```python
from build123d import *

# Parameters (mm, degrees)
F0_W     = 127
F0_H     = 152.4
F0_W_2   = 103
F0_H_2   = 64.5
F1_DEPTH = 6
F2_DEPTH = 2
F3_R     = 3.175


with BuildPart() as f1:
    # F0 (on Top) → F1 (new body)
    with BuildSketch(Plane.XY):
        Rectangle(F0_W, F0_H)
        Rectangle(F0_W_2, F0_H_2, mode=Mode.SUBTRACT)
        Rectangle(F0_W_2, F0_H_2)
    extrude(amount=F1_DEPTH)

    # F0 (on Top) → F2 (cut)
    with BuildSketch(Plane.XY):
        Rectangle(F0_W_2, F0_H_2)
    extrude(amount=F2_DEPTH, mode=Mode.SUBTRACT)

    # F3
    f3_edges = [f1.edges().sort_by_distance(p)[0] for p in [
        (63.5, -76.2, 3),
        (-63.5, -76.2, 3),
        (63.5, 76.2, 3),
        (-63.5, 76.2, 3),
    ]]
    fillet(f3_edges, radius=F3_R)


solid = f1.part
```
Input: part model. Units: mm. Frame: model coordinates. Give positions to 0.01 mm unless a question says otherwise; leave off trailing zeros. Order: outer loops, then holes, each group sorted by start corner. A loop starts at its lowest first (then second) coordinate and runs counter-clockwise, first axis right, second up.
1. Section A-A on z = 1.1. Return the cut outline in (x, y) (3 decimals).
Derived:
outline: (-63.5, -73.025) arc R3.175 ccw to (-60.325, -76.2) - (60.325, -76.2) arc R3.175 ccw to (63.5, -73.025) - (63.5, 73.025) arc R3.175 ccw to (60.325, 76.2) - (-60.325, 76.2) arc R3.175 ccw to (-63.5, 73.025) - close; hole (-51.5, -32.25) - (51.5, -32.25) - (51.5, 32.25) - (-51.5, 32.25) - close
2. Material intervals for L1, parallel to Y at x = -7.5, z = 0.45; L2, parallel to X at y = 29, z = 0.45; L3, parallel to Z at x = -2, y = -12.5, sorted ascending.
Derived:
L1: y = -76.2 to -32.25, 32.25 to 76.2
L2: x = -63.5 to -51.5, 51.5 to 63.5
L3: z = 2 to 6
3. Section B-B on y = -6.5. Return the cut outline in (x, z).
Derived:
outline: (-63.5, 0) - (-51.5, 0) - (-51.5, 2) - (51.5, 2) - (51.5, 0) - (63.5, 0) - (63.5, 6) - (-63.5, 6) - close
4. Mould query, pull axis Y, two halves, no side actions, for faces 1 (the flat face through (-1, 1, 6)), 2 (the flat face through (-1, 76.2, 3)), 3 (the cylindrical face through (62.55, -75.29, 3.04)), 4 (the flat face through (-1, 0, 2)). Classes: released by +Y, released by -Y, zero draft, split by the parting line, or undercut.
Derived:
face 1: zero draft
face 2: released by +Y
face 3: released by -Y
face 4: undercut
5. Section C-C on x = -48. Return the cut outline in (y, z).
Derived:
outline: (-76.2, 0) - (-32.25, 0) - (-32.25, 2) - (32.25, 2) - (32.25, 0) - (76.2, 0) - (76.2, 6) - (-76.2, 6) - close
